```python
from build123d import *

# Parameters (mm, degrees)
SKETCH1_R               = 5.5
SKETCH1_R_2             = 4.999999999999999
BOSS_EXTRUDE1_DEPTH     = 40
FILLET1_R               = 1
FILLET2_R               = 1
CUT_EXTRUDE1_DEPTH      = 41.74923312161882
CUT_EXTRUDE1_DEPTH_BACK = 41.74923312161882
SKETCH2_R               = 1.5000000000000004


with BuildPart() as part:
    # Sketch1 → Boss-Extrude1 (new body)
    with BuildSketch(Plane(origin=(0, 0, 0), x_dir=(1, 0, 0), z_dir=(0, 1, 0))):
        with Locations(Location((0, 0, 0), (0, 0, 270))):
            Circle(SKETCH1_R)
        with Locations(Location((0, 0, 0), (0, 0, 270))):
            Circle(SKETCH1_R_2, mode=Mode.SUBTRACT)
    extrude(amount=BOSS_EXTRUDE1_DEPTH)

    # Fillet1
    # the kernel refuses this fillet: 1 mm, written as the material it takes off along each edge
    with BuildSketch(Plane(origin=(0, 40, 0), x_dir=(-1.8e-16, 0, 1), z_dir=(-1, 0, -1.8e-16))) as fillet1_piece_1:
        with BuildLine():
            CenterArc((5.999999999999999, -0.8660254037844908), FILLET1_R, 119.9999999999984, 60.00000000000159)
            Line((5.500000000000022, -3.553e-14), (5.490000000000022, 0.01732050807565599))
            ThreePointArc((5.490000000000022, 0.01732050807565599), (5.250000000000011, 0.02000000000000313), (4.999999999999999, 0.02000000000000313))
            Line((4.999999999999999, 0.02000000000000313), (4.9799999999999995, 0))
            Line((4.9799999999999995, 0), (4.9799999999999995, -0.8660254037844908))
            Line((4.9799999999999995, -0.8660254037844908), (4.999999999999999, -0.8660254037844908))
        make_face()
    revolve(axis=Axis((0, 40, 0), (0, 1, 0)), mode=Mode.SUBTRACT)

    # Fillet2
    # the kernel refuses this fillet: 1 mm, written as the material it takes off along each edge
    with BuildSketch(Plane(origin=(0, 0, 0), x_dir=(-1.8e-16, 0, 1), z_dir=(-1, 0, -1.8e-16))) as fillet2_piece_1:
        with BuildLine():
            CenterArc((5.999999999999999, 0.866025403784488), FILLET2_R, 180, 60.00000000000148)
            Line((4.999999999999999, 0.866025403784488), (4.9799999999999995, 0.866025403784488))
            Line((4.9799999999999995, 0.866025403784488), (4.9799999999999995, 0))
            Line((4.9799999999999995, 0), (4.999999999999999, -0.02))
            ThreePointArc((4.999999999999999, -0.02), (5.250000000000011, -0.02), (5.4900000000000215, -0.0173205080756525))
            Line((5.4900000000000215, -0.0173205080756525), (5.500000000000021, 3.653e-14))
        make_face()
    revolve(axis=Axis((0, 0, 0), (0, 1, 0)), mode=Mode.SUBTRACT)

    # Sketch2 → Cut-Extrude1 (cut, two sides: drawn at the far end of the back side and taken through both)
    with BuildSketch(Plane(origin=(0, 0, 0), x_dir=(0, 0, -1), z_dir=(1, 0, 0)).offset(-CUT_EXTRUDE1_DEPTH_BACK)):
        with Locations((0, 35)):
            Circle(SKETCH2_R)
    extrude(amount=CUT_EXTRUDE1_DEPTH + CUT_EXTRUDE1_DEPTH_BACK, mode=Mode.SUBTRACT)


solid = part.part
```
Here's how the part is built. I have some questions about the finished solid (model axes, mm). Give positions to 0.01 mm unless a question says otherwise; leave off trailing zeros. Order: outer loops, then holes, each group sorted by start corner. A loop starts at its lowest first (then second) coordinate and runs counter-clockwise, first axis right, second up. Notation, with made-up numbers: M -39.5,52 L -24.5,52 A18 ccw -24.5,67 Z; hole C 21.25,15.5 d6. An arc over 180 degrees is marked long. Use a Markdown table: item, result. Add a question column.
1. I need wall thicknesses on probe 1 along X at (y, z) = (4.5, 0); probe 2 along Z at (x, y) = (3.25, 12.5); probe 3 along X at (y, z) = (10.5, -4.25). Which ranges of each line are inside material? Lowest first, please. Write a range as from..to.
2. For pin 1 Ø2 at (x, y) = (-3.5, 26.5) entering from -Z; pin 2 Ø2.5 at (y, z) = (35, 0) entering from +X; pin 3 Ø4 at (x, y) = (3, 19) entering from +Z; pin 4 Ø2 at (y, z) = (21, 1.5) entering from +X, each with a flat end and sliding along its axis, tell me the tip position at first contact or that it passes through.
3. Suppose I cut it at D-D (y = 22). List the corners of the cut face in (x, z) for me.
4. Suppose I cut it at B-B (y = 35). List the corners of the cut face in (x, z) for me.
5. Suppose I cut it at A-A (x = 0). List the corners of the cut face in (y, z) for me, and give its area (3 significant figures).
6. Suppose I cut it at C-C (z = 0). List the corners of the cut face in (x, y) for me.
Results list:
| question | item | result |
|---|---|---|
| 1 | probe 1 | x = -5.5..-5, 5..5.5 |
| 1 | probe 2 | z = -4.44..-3.8, 3.8..4.44 |
| 1 | probe 3 | x = -3.49..-2.63, 2.63..3.49 |
| 2 | pin 1 | stops at z = -4.9 |
| 2 | pin 2 | passes through |
| 2 | pin 3 | stops at z = 5.41 |
| 2 | pin 4 | stops at x = 5.48 |
| 3 | outline | C 0,0 d11; hole C 0,0 d10 |
| 4 | outline | M -5.29,-1.5 A5.5 ccw 5.29,-1.5 L 4.77,-1.5 A5 cw -4.77,-1.5 Z; M -5.29,1.5 L -4.77,1.5 A5 cw 4.77,1.5 L 5.29,1.5 A5.5 ccw Z |
| 5 | outline | M 0,-5.5 L 40,-5.5 A1 ccw 39.13,-5 L 0.87,-5 A1 ccw Z; M 0,5.5 A1 ccw 0.87,5 L 39.13,5 A1 ccw 40,5.5 Z |
| 5 | area | 39.5 mm² |
| 6 | outline | M -5.5,0 A1 ccw -5,0.87 L -5,33.5 L -5.5,33.5 Z; M -5.5,36.5 L -5,36.5 L -5,39.13 A1 ccw -5.5,40 Z; M 5,0.87 A1 ccw 5.5,0 L 5.5,33.5 L 5,33.5 Z; M 5,36.5 L 5.5,36.5 L 5.5,40 A1 ccw 5,39.13 Z |
